Could you check a few things on this model? Use its own coordinates, in mm. Give positions to 0.01 mm unless a question says otherwise; leave off trailing zeros. Loops run counter-clockwise (first coordinate to the right, second up) from the corner with the lowest first, then second, coordinate; pieces in that order, holes last. Notation, with made-up numbers: M 72,-28 L 122,-28 A25 ccw 122,11 Z; hole C 1,55.5 d1. An arc over 180 degrees is marked long. Return JSON: item names as keys, results as strings. Group by question number.
1. If we section it at B-B (y = 0): Write out the boundary of the cut face in (x, z).
2. If we section it at C-C (z = 10): Write out the boundary of the cut face in (x, y).
3. For pin 1 (0.7 mm diameter, centred on x = 0, y = 2.5, fed in from +Z); pin 2 (2.5 mm diameter, centred on x = -0.5, z = 8, fed in from +Y), each with a flat end and sliding along its axis, tell me the tip position at first contact or that it passes through.
4. If we mould it in two halves opening along Z, with no side actions, what happens to faces 1 (the cylindrical face through (-1.5, -0.64, 9.93)), 2 (the flat face through (-2, 1.65, 10)), 3 (the flat face through (0, 2, 4))? For each: +Z half, -Z half, draft (parallel to the pull), parting line (faces both ways), or undercut.
5. Please list where these lines run through material, in increasing order: line 1 (Z direction, x = 0, y = 0.1); line 2 (Z direction, x = 1, y = 1.5); line 3 (X direction, y = -0.7, z = 10).
6. If we section it at A-A (x = 0): Write out the boundary of the cut face in (y, z).
7. If we section it at D-D (x = -0.75): Write out the boundary of the cut face in (y, z).
```python
from build123d import *

# Parameters (mm, degrees)
SKETCH1_R           = 3
BOSS_EXTRUDE1_DEPTH = 16
CUT_EXTRUDE1_DEPTH  = 12
SKETCH3_R           = 1.5
CUT_EXTRUDE2_DEPTH  = 12


with BuildPart() as part:
    # Sketch1 → Boss-Extrude1 (new body)
    with BuildSketch(Plane.XY):
        Circle(SKETCH1_R)
    extrude(amount=BOSS_EXTRUDE1_DEPTH)

    # Sketch2 → Cut-Extrude1 (cut)
    with BuildSketch(Plane.XY.offset(16)):
        with BuildLine():
            Line((-2.505493963, 1.65), (2.505493963, 1.65))
            ThreePointArc((2.505493963, 1.65), (0, 3), (-2.505493963, 1.65))
        make_face()
    extrude(amount=-CUT_EXTRUDE1_DEPTH, mode=Mode.SUBTRACT)

    # Sketch3 → Cut-Extrude2 (cut)
    with BuildSketch(Plane(origin=(0, 1.65, 0), x_dir=(1, 0, 0), z_dir=(0, 1, 0))):
        with Locations((0, -10)):
            Circle(SKETCH3_R)
    extrude(amount=-CUT_EXTRUDE2_DEPTH, mode=Mode.SUBTRACT)


solid = part.part
```
Answer:
{
 "1": {"outline": "M -3,0 L 3,0 L 3,16 L -3,16 Z; hole C 0,10 d3"},
 "2": {"outline": "M -2.51,1.65 A3 ccw -1.5,-2.6 L -1.5,1.65 Z; M 1.5,-2.6 A3 ccw 2.51,1.65 L 1.5,1.65 Z"},
 "3": {"pin 1": "stops at z = 4", "pin 2": "stops at y = 1.65"},
 "4": {"face 1": "undercut", "face 2": "draft", "face 3": "+Z half"},
 "5": {"line 1": "z = 0 to 8.5, 11.5 to 16", "line 2": "z = 0 to 8.88, 11.12 to 16", "line 3": "x = -2.92 to -1.5, 1.5 to 2.92"},
 "6": {"outline": "M -3,0 L 3,0 L 3,4 L 1.65,4 L 1.65,8.5 L -3,8.5 Z; M -3,11.5 L 1.65,11.5 L 1.65,16 L -3,16 Z"},
 "7": {"outline": "M -2.9,0 L 2.9,0 L 2.9,4 L 1.65,4 L 1.65,8.7 L -2.9,8.7 Z; M -2.9,11.3 L 1.65,11.3 L 1.65,16 L -2.9,16 Z"}
}
